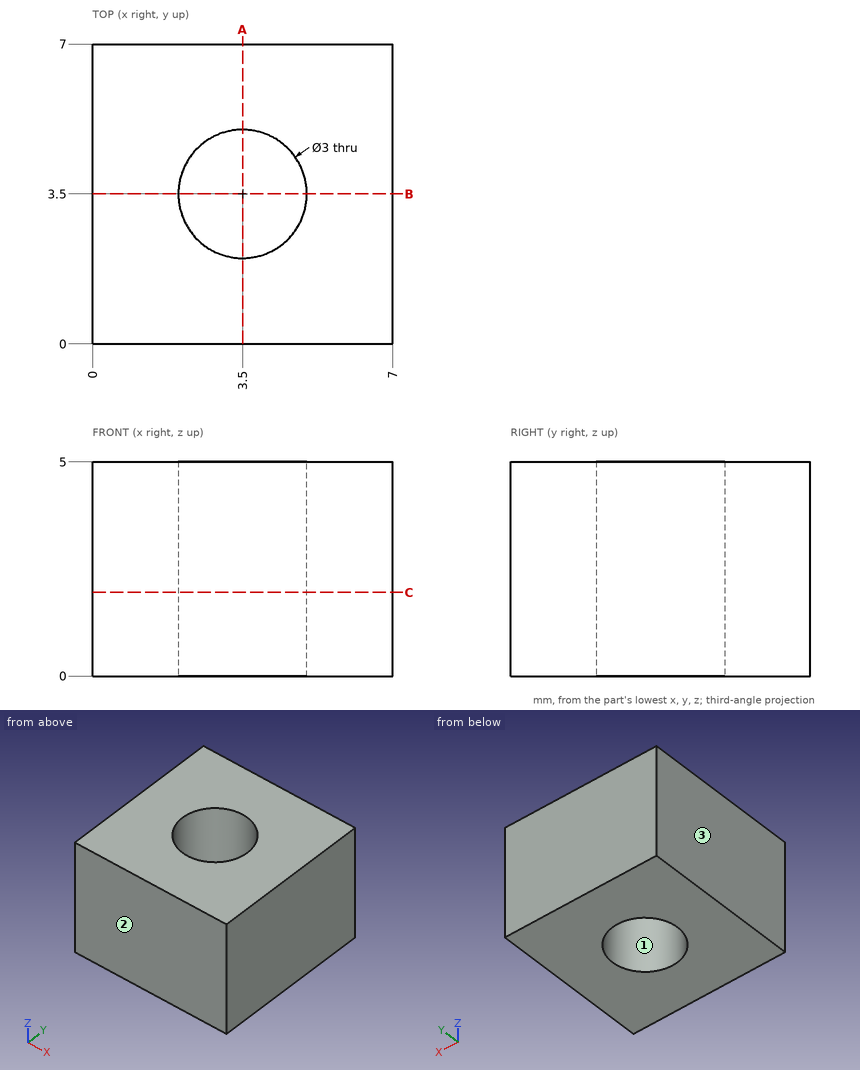
Design review of the part shown in the three views and the two pictorial views. Dimensions are in mm from the part's minimum x, y and z. Coordinates: 2 decimals unless noted, no trailing zeros. Write each loop counter-clockwise with the first axis right and the second up, starting at its lowest first coordinate (ties: lowest second). Pieces come first, ordered by that corner, then holes. Notation, with made-up numbers: (34.5, -33) -> (93.5, -33) arc R28 ccw to (93.5, -15) -> close; hole circle Ø10 at (81, 32.5). An arc over 180 degrees is marked (long way). Answer in a Markdown table with one row per item.
1. Wall thickness on probe 1 along Y at (x, z) = (3.5, 3.9); probe 2 along X at (y, z) = (2.75, 4.25); probe 3 along Y at (x, z) = (4.5, 1.4): over which ranges is each line inside the solid? List them lowest first. Write a range as [from, to].
Answers below:
| item | result |
|---|---|
| probe 1 | y = [0, 2], [5, 7] |
| probe 2 | x = [0, 2.2], [4.8, 7] |
| probe 3 | y = [0, 2.38], [4.62, 7] |
2. Clearance check with a flat-ended pin moving along its axis: pin 1 Ø1.8 at (x, y) = (3.5, 3.5) entering from +Z. State where the tip first meets the part, or that it passes through.
Answers below:
| item | result |
|---|---|
| pin 1 | passes through |
3. We need section A-A, the plane x = 3.5. State the section outline as (y, z) points.
Answers below:
| item | result |
|---|---|
| outline | (0, 0) -> (2, 0) -> (2, 5) -> (0, 5) -> close; (5, 0) -> (7, 0) -> (7, 5) -> (5, 5) -> close |
4. We need section C-C, the plane z = 1.95. State the section outline as (x, y) points, and give its area (3 significant figures).
Answers below:
| item | result |
|---|---|
| outline | (0, 0) -> (7, 0) -> (7, 7) -> (0, 7) -> close; hole circle Ø3 at (3.5, 3.5) |
| area | 41.9 mm^2 |
5. Draft analysis for pull direction X (two halves, no side actions). For the marked faces 1, 2 and 3, state which applies: +X half, -X half, draft (parallel to the pull), parting line (faces both ways), or undercut.
Answers below:
| item | result |
|---|---|
| face 1 | undercut |
| face 2 | draft |
| face 3 | -X half |
